Here's the drawing with two shaded views (mm, measured from the low corner). I have some questions. Coordinates: 2 decimals unless noted, no trailing zeros. Loops run counter-clockwise (first coordinate to the right, second up) from the corner with the lowest first, then second, coordinate; pieces in that order, holes last. Notation, with made-up numbers: M 21,10.5 L 73,10.5 A28 ccw 73,45.5 Z; hole C 48,-20 d2. An arc over 180 degrees is marked long. Use one line per item in the form item = value. Start each with the question number.
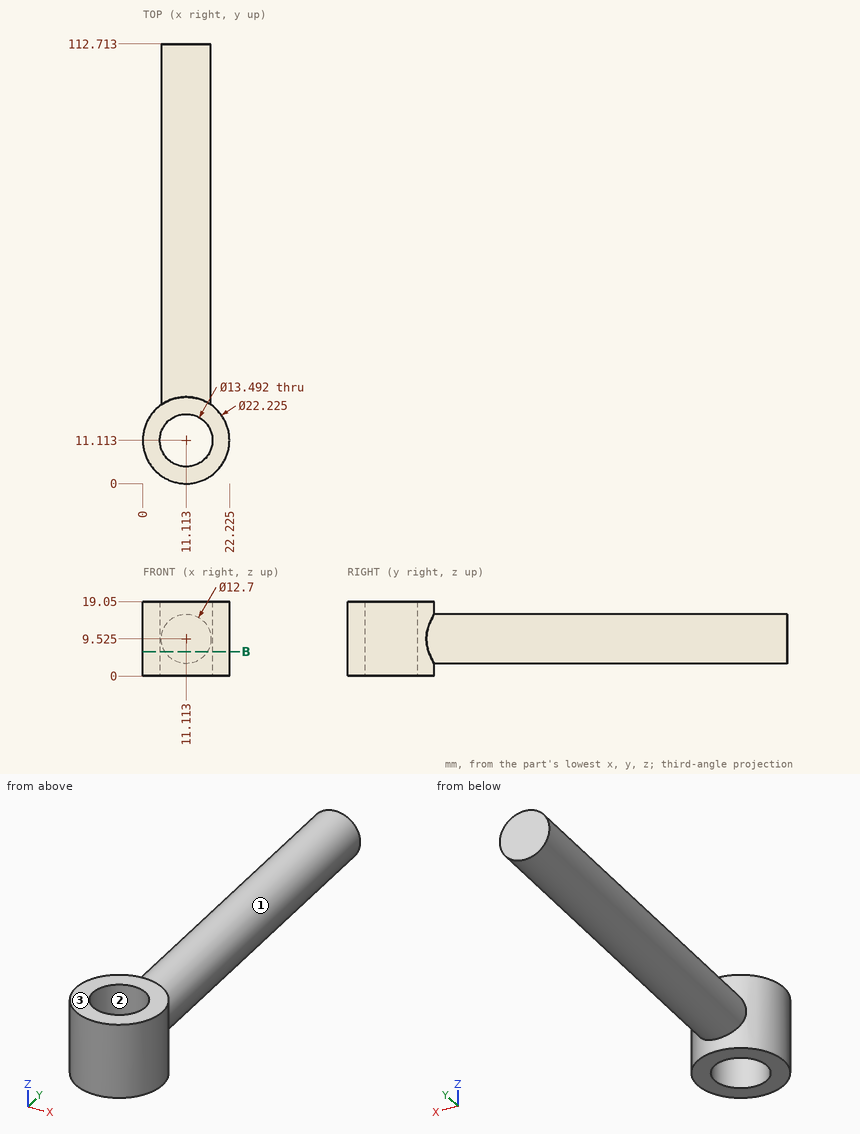
Item 1: I want a section at B-B (z = 6.25). Write out the boundary of the cut face in (x, y) (1 decimal), plus the area to 3 significant figures.
Item 2: Thinking about a two-plate mould opening in X: for the marked faces 1, 2 and 3, which applies, pulls with the +X half, pulls with the -X half, needs draft (parallel to the pull), parting line crosses it, or undercut?
Item 3: Please list where these lines run through material, in increasing order: line 1 along Y through (x, z) = (11.25, 1.5) (1 decimal); line 2 along Y through (x, z) = (13, 6.25) (1 decimal); line 3 along X through (y, z) = (12.5, 10.25) (1 decimal).
Item 4: I'm going to push flat-ended pins straight in: P1, Ø1.5, axis at x = 17, y = 88.5, coming from the +Z side (1 decimal); P2, Ø3, axis at x = 6.5, y = 60, coming from the -Z side; P3, Ø1.5, axis at x = 5.5, z = 4, coming from the +Y side (1 decimal). Where does each tip first touch, or does it pass through?
Worked answers:
q1.outline = M 5.7,20.8 A11.1 ccw long 16.6,20.8 L 16.6,112.7 L 5.7,112.7 Z; hole C 11.1,11.1 d13.5
q1.area = 1,230 mm²
q2.face_1 = parting line crosses it
q2.face_2 = undercut
q2.face_3 = needs draft
q3.line_1 = 0 to 4.4, 17.9 to 22.2
q3.line_2 = 0.2 to 4.6, 17.6 to 112.7
q3.line_3 = 0.1 to 4.5, 17.7 to 22.1
q4.P1 = 13.3
q4.P2 = 3.99
q4.P3 = 21.1
